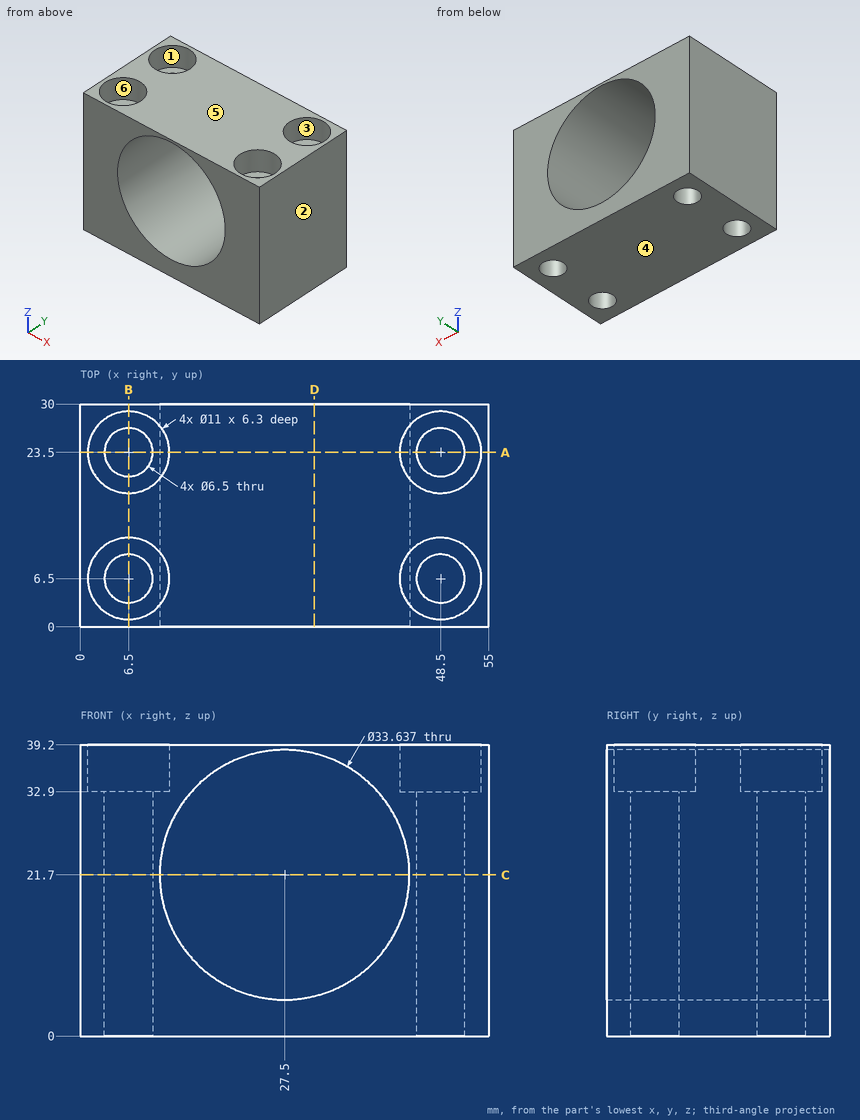
Can you work these out from the drawing? Everything is in mm from the part's minimum corner. A direction names the side the tool comes from. Round coordinates to 2 decimals unless told otherwise and drop trailing zeros. Order: outer loops, then holes, each group sorted by start corner. A loop starts at its lowest first (then second) coordinate and runs counter-clockwise, first axis right, second up.
(1) If we section it at B-B (x = 6.5): Please give me the cut outline in (y, z).
Results are:
outline: (0, 0) - (3.25, 0) - (3.25, 32.9) - (1, 32.9) - (1, 39.2) - (0, 39.2) - close; (9.75, 0) - (20.25, 0) - (20.25, 32.9) - (18, 32.9) - (18, 39.2) - (12, 39.2) - (12, 32.9) - (9.75, 32.9) - close; (26.75, 0) - (30, 0) - (30, 39.2) - (29, 39.2) - (29, 32.9) - (26.75, 32.9) - close
(2) If we section it at D-D (x = 31.5): Please give me the cut outline in (y, z) (1 decimal).
Results are:
outline: (0, 0) - (30, 0) - (30, 5.4) - (0, 5.4) - close; (0, 38) - (30, 38) - (30, 39.2) - (0, 39.2) - close
(3) If I drill on L1, parallel to Y at x = 48.5, z = 8; L2, parallel to X at y = 23.25, z = 24; L3, parallel to X at y = 27, z = 21.5, over which ranges is the centre line in solid material (lowest first)?
Results are:
L1: y = 0 to 3.25, 9.75 to 20.25, 26.75 to 30
L2: x = 0 to 3.26, 9.74 to 10.84, 44.16 to 45.26, 51.74 to 55
L3: x = 0 to 10.68, 44.32 to 55
(4) We'd pull the mould along X, two halves only. Please class the marked faces 1, 2, 3 and 4: +X half, -X half, draft (parallel to the pull), parting line (faces both ways), or undercut.
Results are:
face 1: undercut
face 2: +X half
face 3: undercut
face 4: draft
(5) On a 3-axis mill with a long thin cutter (end or side, diameter ignored), from which of +Z, -Z, +X, -X, +Y, -Y can I reach the whole of each face in a straight line? I mean the marked faces 5 and 6. Say none if no direction works.
Results are:
face 5: +Z, +X, -X, +Y, -Y
face 6: +Z
(6) If we section it at C-C (z = 21.7): Please give me the cut outline in (x, y).
Results are:
outline: (0, 0) - (10.68, 0) - (10.68, 30) - (0, 30) - close; (44.32, 0) - (55, 0) - (55, 30) - (44.32, 30) - close; hole circle Ø6.5 at (6.5, 6.5); hole circle Ø6.5 at (6.5, 23.5); hole circle Ø6.5 at (48.5, 6.5); hole circle Ø6.5 at (48.5, 23.5)
(7) I'm going to push a flat-ended pin straight in: pin 1 (8.5 mm diameter, centred on x = 48.5, y = 6.5, fed in from +Z). Where does the tip first touch, or does it pass through?
Results are:
pin 1: stops at z = 32.9
(8) If we section it at A-A (y = 23.5): Please give me the cut outline in (x, z), plus the area to 3 significant figures.
Results are:
outline: (0, 0) - (3.25, 0) - (3.25, 32.9) - (1, 32.9) - (1, 39.2) - (0, 39.2) - close; (9.75, 0) - (45.25, 0) - (45.25, 32.9) - (43, 32.9) - (43, 39.2) - (12, 39.2) - (12, 32.9) - (9.75, 32.9) - close; (51.75, 0) - (55, 0) - (55, 39.2) - (54, 39.2) - (54, 32.9) - (51.75, 32.9) - close; hole circle Ø33.64 at (27.5, 21.7)
area: 701 mm2
